```python
from build123d import *

# Parameters (mm, degrees)
F1_DEPTH     = 14
F2_R         = 2
F3_W         = 4.692493906
F3_H         = 14
F4_DEPTH     = 60
F5_SIZE      = 8
F6_R         = 0.3
F7_T1_DEPTH  = 14
F7_T4_ANGLE  = 90
F7_T6_ANGLE  = 90
F7_T8_ANGLE  = 90
F7_T10_ANGLE = 90


# Not quite as in the source:
# - a fillet or chamfer that OpenCascade refuses, or shapes differently, is made with other operations: its cross-section is extruded or revolved along the edge and cut away or added
# - a feature names something its author has since deleted; it is built from what else it names


with BuildPart() as f1:
    # F0 (on Top) → F1 (new body)
    with BuildSketch(Plane.XY):
        Polygon((0, 27), (0, 0), (-0.7, -4.7870394774), (7, -4.7870394774), (7, 35), (-13, 35), (-13, -4.7870394774), (-5.3, -4.7870394774), (-6, 0), (-6, 27), align=None)
    extrude(amount=F1_DEPTH)

    # F2
    f2_edges = [f1.edges().sort_by_distance(p)[0] for p in [
        (-13, 35, 7),
        (-13, -4.787039, 7),
        (0, 27, 7),
        (0, 0, 7),
        (7, 35, 7),
        (-6, 0, 7),
        (-6, 27, 7),
    ]]
    fillet(f2_edges, radius=F2_R)

    # F3 (on face) → F4 (join)
    with BuildSketch(Plane(origin=(0, 0, 0), x_dir=(-0.1446894238, -0.9894771198, 0), z_dir=(-0.9894771198, 0.1446894238, 0))):
        with Locations((2.4917016782, 7)):
            Rectangle(F3_W, F3_H)
    extrude(amount=-F4_DEPTH)

    # F5
    f5_edges = [f1.edges().sort_by_distance(p)[0] for p in [
        (7, -1.170599, 7),
    ]]
    chamfer(f5_edges, length=F5_SIZE)

    # F6
    f6_edges = [f1.edges().sort_by_distance(p)[0] for p in [
        (37.131699, -5.576702, 14),
        (10.957908, 2.250644, 14),
        (59.008104, -11.146847, 14),
        (7, 19.914701, 14),
        (28.984314, -9.127722, 14),
        (6.414214, 34.414214, 14),
        (-0.360523, -2.465482, 14),
        (-3, 35, 14),
        (-0.005268, 0.000383, 14),
        (-12.414214, 34.414214, 14),
        (0, 12.572727, 14),
        (-13, 15.10648, 14),
        (-0.585786, 26.414214, 14),
        (-12.414214, -4.201253, 14),
        (-3, 27, 14),
        (-8.15, -4.787039, 14),
        (-5.414214, 26.414214, 14),
        (-5.639477, -2.465482, 14),
        (-6, 12.572727, 14),
        (-5.994732, 0.000383, 14),
        (37.131699, -5.576702, 0),
        (10.957908, 2.250644, 0),
        (59.008104, -11.146847, 0),
        (7, 19.914701, 0),
        (28.984314, -9.127722, 0),
        (6.414214, 34.414214, 0),
        (-0.360523, -2.465482, 0),
        (-3, 35, 0),
        (-0.005268, 0.000383, 0),
        (-12.414214, 34.414214, 0),
        (0, 12.572727, 0),
        (-13, 15.10648, 0),
        (-0.585786, 26.414214, 0),
        (-12.414214, -4.201253, 0),
        (-3, 27, 0),
        (-8.15, -4.787039, 0),
        (-5.414214, 26.414214, 0),
        (-5.639477, -2.465482, 0),
        (-6, 12.572727, 0),
        (-5.994732, 0.000383, 0),
    ]]
    fillet(f6_edges, radius=F6_R)

    # F7: fillet of radius 1 on 2 edges, made by hand

    # F7_s2 → F7_t1 (cut)
    with BuildSketch(Plane.XY):
        with BuildLine():
            ThreePointArc((58.3581043085, -8.6806001289), (59.0153917386, -9.0727221402), (59.2028920045, -9.8147666726))
            Line((59.2028920045, -9.8147666726), (59.3475814283, -8.8252895527))
            Line((59.3475814283, -8.8252895527), (58.3581043085, -8.6806001289))
        make_face()
        with BuildLine():
            ThreePointArc((58.8133166125, -12.4789277878), (58.4211946012, -13.136215218), (57.6791500689, -13.3237154838))
            Line((57.6791500689, -13.3237154838), (58.6686271887, -13.4684049076))
            Line((58.6686271887, -13.4684049076), (58.8133166125, -12.4789277878))
        make_face()
    extrude(amount=F7_T1_DEPTH, mode=Mode.SUBTRACT)

    # F7_s3 → F7_t4 (revolve, cut)
    with BuildSketch(Plane(origin=(-0.5553105762, -3.7975623576, 0), x_dir=(0, 0, 1), z_dir=(0.1446894238, 0.9894771198, 0))):
        with BuildLine():
            ThreePointArc((0, 59.7), (0.0878679656, 59.9121320344), (0.3, 60))
            Line((0.3, 60), (0, 60))
            Line((0, 60), (0, 59.7))
        make_face()
    revolve(axis=Axis((57.8238394927, -12.334238364, 0), (0, 0, -1)), revolution_arc=F7_T4_ANGLE, mode=Mode.SUBTRACT)

    # F7_s5 → F7_t6 (revolve, cut)
    with BuildSketch(Plane(origin=(58.3791500689, -8.5366760064, 0), x_dir=(0, 0, 1), z_dir=(-0.9894771198, 0.1446894238, 0))):
        with BuildLine():
            ThreePointArc((14, -4.5379486312), (13.9121320344, -4.7500806655), (13.7, -4.8379486312))
            Line((13.7, -4.8379486312), (14, -4.8379486312))
            Line((14, -4.8379486312), (14, -4.5379486312))
        make_face()
    revolve(axis=Axis((57.8238394927, -12.334238364, 14), (0, 0, 1)), revolution_arc=F7_T6_ANGLE, mode=Mode.SUBTRACT)

    # F7_s7 → F7_t8 (revolve, cut)
    with BuildSketch(Plane(origin=(-0.1657351842, -1.1334012423, 0), x_dir=(0, 0, 1), z_dir=(-0.1446894238, -0.9894771198, 0))):
        with BuildLine():
            ThreePointArc((14, -59.7), (13.9121320344, -59.9121320344), (13.7, -60))
            Line((13.7, -60), (14, -60))
            Line((14, -60), (14, -59.7))
        make_face()
    revolve(axis=Axis((58.2134148846, -9.6700772487, 14), (0, 0, 1)), revolution_arc=F7_T8_ANGLE, mode=Mode.SUBTRACT)

    # F7_s9 → F7_t10 (revolve, cut)
    with BuildSketch(Plane(origin=(58.3791500689, -8.5366760064, 0), x_dir=(0, 0, 1), z_dir=(-0.9894771198, 0.1446894238, 0))):
        with BuildLine():
            ThreePointArc((0, -0.4454547252), (0.0878679656, -0.2333226908), (0.3, -0.1454547252))
            Line((0.3, -0.1454547252), (0, -0.1454547252))
            Line((0, -0.1454547252), (0, -0.4454547252))
        make_face()
    revolve(axis=Axis((58.2134148846, -9.6700772487, 0), (0, 0, -1)), revolution_arc=F7_T10_ANGLE, mode=Mode.SUBTRACT)


solid = f1.part
```
Check sheet for the modelled part. Datum: model origin and axes. Units: mm. A direction names the side the tool comes from. Round coordinates to 2 decimals unless told otherwise and drop trailing zeros. Loops run counter-clockwise (first coordinate to the right, second up) from the corner with the lowest first, then second, coordinate; pieces in that order, holes last. Notation, with made-up numbers: (-23.5, 18.5) -> (29.5, 18.5) arc R28 cw to (29.5, 37.5) -> close; hole circle Ø1 at (-9.5, 87.5). An arc over 180 degrees is marked (long way). Write item = value, one per line. Start each with the question number.
1) Gauge pin test, flat ends, axial feed: pin 1 Ø1 at (x, z) = (49.5, 7) entering from +Y; pin 2 Ø4 at (x, y) = (22, -3.5) entering from +Z; pin 3 Ø2 at (x, z) = (-3.5, 7) entering from -Y; pin 4 Ø5 at (y, z) = (9, 12) entering from +X. Record the tip position at first contact, or that the pin passes through.
2) Sectioned sample at A-A, the plane y = 15.5. Record the cut outline in (x, z).
3) Release check for a two-part mould opening along X. For faces 1 (the cylindrical face through (-12.4, 34.43, 7.09)), 2 (the flat face through (7, 6, 0)), 3 (the cylindrical face through (10.95, 2.13, 13.91)), 4 (the flat face through (-6, 12, 7)) record: released by +X, released by -X, zero draft, split by the parting line, or undercut.
4) Thickness scan on probe 1 along X at (y, z) = (23.5, 4.5); probe 2 along Y at (x, z) = (-6.5, 13); probe 3 along X at (y, z) = (5, 4.5). Record the ranges inside material, lowest first.
5) Set-up check for faces 5 (the flat face through (-8, -4.787, 7)), 6 (the cylindrical face through (10.95, 2.13, 0.09)), 7 (the flat face through (7, 20, 7)), 8 (the cylindrical face through (-0.57, 26.4, 7.09)): record each of +Z, -Z, +X, -X, +Y, -Y from which the full face is reachable in a straight line by a thin tool's end or side.
6) Sectioned sample at B-B, the plane z = 10.5. Record the cut outline in (x, y).
Results are:
q1.pin_1 = -7.31
q1.pin_2 = 14
q1.pin_3 = 26.94
q1.pin_4 = 7.28
q2.outline = (-13, 0.3) arc R0.3 ccw to (-12.7, 0) -> (-6.3, 0) arc R0.3 ccw to (-6, 0.3) -> (-6, 13.7) arc R0.3 ccw to (-6.3, 14) -> (-12.7, 14) arc R0.3 ccw to (-13, 13.7) -> close; (0, 0.3) arc R0.3 ccw to (0.3, 0) -> (6.7, 0) arc R0.3 ccw to (7, 0.3) -> (7, 13.7) arc R0.3 ccw to (6.7, 14) -> (0.3, 14) arc R0.3 ccw to (0, 13.7) -> close
q3.face_1 = released by -X
q3.face_2 = zero draft
q3.face_3 = released by +X
q3.face_4 = undercut
q4.probe_1 = -13 to -6, 0 to 7
q4.probe_2 = -4.79 to 35
q4.probe_3 = -13 to -6, 0 to 8.58
q5.face_5 = +Z, -Z, -X, -Y
q5.face_6 = -Z, +X, +Y
q5.face_7 = +Z, -Z, +X, +Y
q5.face_8 = +Z, -Z
q6.outline = (-13, -2.79) arc R2 ccw to (-11, -4.79) -> (-5.3, -4.79) -> (-5.98, -0.14) arc R2 cw to (-6, 0.15) -> (-6, 25) arc R2 cw to (-4, 27) -> (-2, 27) arc R2 cw to (0, 25) -> (0, 0.15) arc R2 cw to (-0.02, -0.14) -> (-0.7, -4.79) -> (57.68, -13.32) arc R1 ccw to (58.81, -12.48) -> (59.2, -9.81) arc R1 ccw to (58.36, -8.68) -> (14.92, -2.33) -> (7, 6.83) -> (7, 33) arc R2 ccw to (5, 35) -> (-11, 35) arc R2 ccw to (-13, 33) -> close
